```python
from build123d import *

# Parameters (mm, degrees)
SKETCH2_R           = 1.1303
BOSS_EXTRUDE1_DEPTH = 25.4
SKETCH3_R           = 1.905
BOSS_EXTRUDE2_DEPTH = 5.08
CUT_EXTRUDE1_DEPTH  = 5.08


with BuildPart() as part:
    # Sketch2 → Boss-Extrude1 (new body)
    with BuildSketch(Plane(origin=(0, 0, 0), x_dir=(0, 0, -1), z_dir=(1, 0, 0))):
        Circle(SKETCH2_R)
    extrude(amount=-BOSS_EXTRUDE1_DEPTH)

    # Sketch3 → Boss-Extrude2 (add)
    with BuildSketch(Plane(origin=(0, 0, 0), x_dir=(0, 0, -1), z_dir=(1, 0, 0))):
        Circle(SKETCH3_R)
    extrude(amount=BOSS_EXTRUDE2_DEPTH)

    # Sketch4 → Cut-Extrude1 (cut)
    with BuildSketch(Plane(origin=(5.08, 0, 0), x_dir=(0, 0, -1), z_dir=(1, 0, 0))):
        with BuildLine():
            Line((-1.495366573, 1.18021346), (1.495366573, 1.18021346))
            ThreePointArc((1.495366573, 1.18021346), (0, 1.905), (-1.495366573, 1.18021346))
        make_face()
    extrude(amount=-CUT_EXTRUDE1_DEPTH, mode=Mode.SUBTRACT)


solid = part.part
```
Source: CAD feature listing. Evaluate the final solid. Frame: model axes, mm. A direction names the side the tool comes from. Give positions to 0.01 mm unless a question says otherwise; leave off trailing zeros. Loops run counter-clockwise (first coordinate to the right, second up) from the corner with the lowest first, then second, coordinate; pieces in that order, holes last. Notation, with made-up numbers: (45.5, -32) -> (63.5, -32) arc R24 cw to (63.5, -3) -> close; hole circle Ø9 at (1.5, 62). An arc over 180 degrees is marked (long way). Use a Markdown table: item, result. Add a question column.
(1) Section query C-C (x = -6.5). Output: boundary loops of the cut face in (y, z).
(2) Section query A-A (z = 0). Output: boundary loops of the cut face in (x, y) (3 decimals).
(3) Section query B-B (y = 0). Output: boundary loops of the cut face in (x, z) (3 decimals), then the cut area to 3 significant figures.
(4) Access query for faces 1 (the face through (-25.4, 0, 0)), 2 (the face through (-12.522, -1.103, 0.245)). Directions: +Z, -Z, +X, -X, +Y, -Y. A direction counts if a zero-diameter tool reaches every point of the face in a straight line with its end or side. Return the directions, or none.
(5) Ray query, line 1 (X direction, y = -0.3, z = -1.4); line 2 (Y direction, x = -18, z = 0.85); line 3 (Z direction, x = 0.5, y = -0.45). Return the intervals inside material, ascending.
Checked values:
| question | item | result |
|---|---|---|
| 1 | outline | circle Ø2.26 at (0, 0) |
| 2 | outline | (-25.4, -1.13) -> (0, -1.13) -> (0, -1.905) -> (5.08, -1.905) -> (5.08, 1.18) -> (0, 1.18) -> (0, 1.13) -> (-25.4, 1.13) -> close |
| 3 | outline | (-25.4, -1.13) -> (0, -1.13) -> (0, -1.905) -> (5.08, -1.905) -> (5.08, 1.905) -> (0, 1.905) -> (0, 1.13) -> (-25.4, 1.13) -> close |
| 3 | area | 76.8 mm^2 |
| 4 | face 1 | +Z, -Z, -X, +Y, -Y |
| 4 | face 2 | -X |
| 5 | line 1 | 0 to 5.08 |
| 5 | line 2 | -0.75 to 0.75 |
| 5 | line 3 | -1.85 to 1.85 |
